Check sheet for the modelled part. Datum: model origin and axes. Units: mm. A direction names the side the tool comes from. Round coordinates to 2 decimals unless told otherwise and drop trailing zeros. Write each loop counter-clockwise with the first axis right and the second up, starting at its lowest first coordinate (ties: lowest second). Pieces come first, ordered by that corner, then holes. Notation, with made-up numbers: (-8.75, 60) -> (4.25, 60) arc R33 ccw to (4.25, 98) -> close; hole circle Ø5 at (32, 21). An arc over 180 degrees is marked (long way). Write item = value, one per line.
from build123d import *

# Parameters (mm, degrees)
SKETCH_W             = 89
SKETCH_H             = 4.5
PAD_DEPTH            = 125
SKETCH001_W          = 76.5
SKETCH001_H          = 76.5
POCKET_DEPTH         = 3.5
SKETCH002_W          = 70
SKETCH002_H          = 70
POCKET001_DEPTH      = 1.001
POCKET001_DEPTH_BACK = 3.501
SKETCH003_W          = 89
SKETCH003_H          = 15
PAD001_DEPTH         = 5
CHAMFER_SIZE         = 2


with BuildPart() as part:
    # Sketch → Pad (new body)
    with BuildSketch(Plane.XZ):
        Rectangle(SKETCH_W, SKETCH_H)
    extrude(amount=-PAD_DEPTH)

    # Sketch001 (on Face2 of Pad) → Pocket (cut)
    with BuildSketch(Plane.XY.offset(2.25)):
        with Locations((0, 65.75)):
            Rectangle(SKETCH001_W, SKETCH001_H)
    extrude(amount=-POCKET_DEPTH, mode=Mode.SUBTRACT)

    # Sketch002 (on Face11 of Pocket) → Pocket001 (cut, two sides)
    with BuildSketch(Plane.XY.offset(-1.25)) as pocket001_sk:
        with Locations((0, 65.75)):
            Rectangle(SKETCH002_W, SKETCH002_H)
    extrude(amount=-POCKET001_DEPTH, mode=Mode.SUBTRACT)
    extrude(pocket001_sk.sketch, amount=POCKET001_DEPTH_BACK, mode=Mode.SUBTRACT)

    # Sketch003 (on Face4 of Pocket001) → Pad001 (join)
    with BuildSketch(Plane.XZ):
        with Locations((0, 5.25)):
            Rectangle(SKETCH003_W, SKETCH003_H)
    extrude(amount=PAD001_DEPTH)

    # Chamfer
    chamfer_edges = [part.edges().sort_by_distance(p)[0] for p in [
        (0, -5, 12.75),
        (44.5, -2.5, 12.75),
        (0, 0, 12.75),
        (-44.5, -2.5, 12.75),
        (-44.5, -5, 5.25),
        (44.5, -5, 5.25),
    ]]
    chamfer(chamfer_edges, length=CHAMFER_SIZE)


solid = part.part
(1) Material ranges on L1, parallel to X at y = 78, z = 0.25; L2, parallel to Y at x = 33.5, z = 0.75; L3, parallel to Y at x = -3, z = -1.5, recorded low to high. Write a range as [from, to].
Worked answers:
L1 = [-44.5, -38.25], [38.25, 44.5]
L2 = [-5, 27.5], [104, 125]
L3 = [-5, 30.75], [100.75, 125]
(2) Release check for a two-part mould opening along Y. For faces 1 (the flat face through (-3, 29, -1.25)), 2 (the flat face through (-1, 20, 2.25)), 3 (the flat face through (38.25, 65, 1)), 4 (the flat face through (-1, -5, 4)) record: pulls with the +Y half, pulls with the -Y half, needs draft (parallel to the pull), parting line crosses it, or undercut.
Worked answers:
face_1 = undercut
face_2 = needs draft
face_3 = undercut
face_4 = pulls with the -Y half
(3) Sectioned sample at D-D on y = 105.5. Enter the section's corners in (x, z).
Worked answers:
outline = (-44.5, -2.25) -> (44.5, -2.25) -> (44.5, 2.25) -> (-44.5, 2.25) -> close
(4) Go/stop test with a flat-tipped pin: P1, Ø4, axis at x = 18.5, z = 5.5, coming from the +Y side. Record where the tip stops, or that it passes through.
Worked answers:
P1 = 0
(5) Sectioned sample at C-C on z = 7.5. Enter the section's corners in (x, y).
Worked answers:
outline = (-44.5, -3) -> (-42.5, -5) -> (42.5, -5) -> (44.5, -3) -> (44.5, 0) -> (-44.5, 0) -> close
(6) Sectioned sample at B-B on y = 53. Enter the section's corners in (x, z).
Worked answers:
outline = (-44.5, -2.25) -> (-35, -2.25) -> (-35, -1.25) -> (-38.25, -1.25) -> (-38.25, 2.25) -> (-44.5, 2.25) -> close; (35, -2.25) -> (44.5, -2.25) -> (44.5, 2.25) -> (38.25, 2.25) -> (38.25, -1.25) -> (35, -1.25) -> close
(7) Access from +Z, -Z, +X, -X, +Y, -Y to the whole of each face (thin tool, end or side, straight path). Record for faces 5 (the flat face through (-1, 104, 1)), 6 (the flat face through (-1, 0, 7)), 7 (the flat face through (-1, 125, 0)).
Worked answers:
face_5 = +Z
face_6 = +Z, +X, -X, +Y
face_7 = +Z, -Z, +X, -X, +Y
(8) Sectioned sample at A-A on x = -19.5. Enter the section's corners in (y, z), then the cut area to 3 significant figures.
Worked answers:
outline = (-5, -2.25) -> (30.75, -2.25) -> (30.75, -1.25) -> (27.5, -1.25) -> (27.5, 2.25) -> (0, 2.25) -> (0, 10.75) -> (-2, 12.75) -> (-3, 12.75) -> (-5, 10.75) -> close; (100.75, -2.25) -> (125, -2.25) -> (125, 2.25) -> (104, 2.25) -> (104, -1.25) -> (100.75, -1.25) -> close
area = 296 mm²
